from build123d import *

# Parameters (mm, degrees)
PAD_DEPTH          = 56
SKETCH005_R        = 1.25
POCKET_DEPTH       = 236.830052
POCKET_DEPTH_BACK  = 294.830052
POCKET001_DEPTH    = 237.830052
POLARPATTERN_COUNT = 6


with BuildPart() as part:
    # Sketch → Revolution002 (revolve)
    with BuildSketch(Plane.XZ):
        with BuildLine():
            Line((12, 0), (12, 58))
            Line((12, 58), (36.5, 58))
            Line((36.5, 55), (36.5, 58))
            Line((31, 55), (36.5, 55))
            Line((31, 4.25), (31, 55))
            Line((36.5, 4.25), (31, 4.25))
            Line((36.5, 1.25), (36.5, 4.25))
            Line((36.5, 1.25), (17, 1.25))
            Line((17, 1.25), (17, 0.5))
            ThreePointArc((16.5, 0), (16.853553, 0.146447), (17, 0.5))
            Line((16.5, 0), (12, 0))
        make_face()
    revolve(axis=Axis((0, 0, 0), (0, 0, 1)))

    # Sketch004 → Pad (new body)
    with BuildSketch(Plane.XY.offset(58)):
        with BuildLine():
            ThreePointArc((30.765894, -3.802601), (31, 0), (30.765894, 3.802601))
            ThreePointArc((30.765894, 3.802601), (30.872245, 3.491837), (31.094507, 3.25))
            Line((31.907923, 2.668318), (31.094507, 3.25))
            ThreePointArc((32.765894, 1), (32.538832, 1.938003), (31.907923, 2.668318))
            Line((32.765894, 1), (32.765894, -1))
            ThreePointArc((31.907923, -2.668318), (32.538832, -1.938003), (32.765894, -1))
            Line((31.907923, -2.668318), (31.094507, -3.25))
            ThreePointArc((31.094507, -3.25), (30.872245, -3.491837), (30.765894, -3.802601))
        make_face()
    pad = extrude(amount=-PAD_DEPTH)

    # Sketch005 → Pocket (cut, two sides)
    with BuildSketch(Plane.XY) as pocket_sk:
        with Locations((31.25, 0)):
            Circle(SKETCH005_R)
    pocket = extrude(amount=-POCKET_DEPTH, mode=Mode.SUBTRACT) + extrude(pocket_sk.sketch, amount=POCKET_DEPTH_BACK, mode=Mode.SUBTRACT)

    # Sketch006 → Pocket001 (cut, through all)
    with BuildSketch(Plane.XY.offset(57)):
        with BuildLine():
            ThreePointArc((15.210029, 5.719923), (14.056331, 8.153652), (12.516493, 10.363393))
            ThreePointArc((12.41083, 12.132293), (12.17453, 11.230572), (12.516493, 10.363393))
            Line((20.118158, 24.097608), (12.41083, 12.132293))
            ThreePointArc((23.174899, 24.466591), (21.559851, 25.000154), (20.118158, 24.097608))
            ThreePointArc((32.743937, 7.970232), (29.150669, 16.90942), (23.174899, 24.466591))
            ThreePointArc((30.906067, 5.5), (32.405281, 6.303385), (32.743937, 7.970232))
            Line((16.693075, 4.75), (30.906067, 5.5))
            ThreePointArc((15.210029, 5.719923), (15.793016, 4.992554), (16.693075, 4.75))
        make_face()
    pocket001 = extrude(amount=POCKET001_DEPTH, mode=Mode.SUBTRACT)

    # PolarPattern: Pad, Pocket, Pocket001 ×6 about axis
    polarpattern_axis = Axis((0, 0, 58), (0, 0, 1))
    for i in range(1, POLARPATTERN_COUNT):
        add(pad.rotate(polarpattern_axis, i * 360 / POLARPATTERN_COUNT))
        add(pocket.rotate(polarpattern_axis, i * 360 / POLARPATTERN_COUNT), mode=Mode.SUBTRACT)
        add(pocket001.rotate(polarpattern_axis, i * 360 / POLARPATTERN_COUNT), mode=Mode.SUBTRACT)


solid = part.part
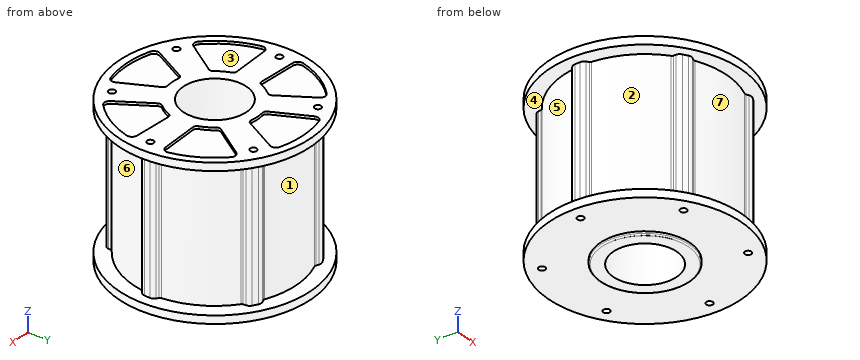
Read the model definition and answer for the solid it produces. Units are mm, in the model's axes. Face numbers are marked on the shaded views. A direction names the side the tool comes from. Coordinates: 2 decimals unless noted, no trailing zeros. Loops run counter-clockwise (first coordinate to the right, second up) from the corner with the lowest first, then second, coordinate; pieces in that order, holes last. Notation, with made-up numbers: (14.5, 14) - (58.5, 14) arc R7 ccw to (58.5, 18) - close; hole circle Ø6 at (45.25, -1). An arc over 180 degrees is marked (long way). Answer in a Markdown table with one row per item.
Q1. Straight lines are drawn through the part: line 1 along X through (y, z) = (-27, 39); line 2 along Z through (x, y) = (-21, -3); line 3 along Z through (x, y) = (18, 12). For each, find the intervals that lie inside material, in ascending order. Write a range as [from, to].
Here are the results:
| item | result |
|---|---|
| line 1 | x = [-18.07, -16.87], [-14.38, 14.38], [16.87, 18.07] |
| line 2 | z = [1.25, 58] |
| line 3 | z = [1.25, 57] |
Q2. The mould has two halves that part along X. Classify the marked faces 5, 6 and 7: pulls with the +X half, pulls with the -X half, needs draft (parallel to the pull), parting line crosses it, or undercut.
Here are the results:
| item | result |
|---|---|
| face 5 | pulls with the -X half |
| face 6 | pulls with the +X half |
| face 7 | undercut |
Q3. Given P1, Ø10, axis at y = 17.5, z = 37, coming from the +X side; P2, Ø1.5, axis at x = 31.25, y = 0, coming from the +Z side; P3, Ø2, axis at y = 0, z = 36, coming from the +X side; P4, Ø1, axis at x = 17, z = 18, coming from the +Y side, each flat-ended and moving along its own axis, determine where each tip first touches the part or whether it passes through.
Here are the results:
| item | result |
|---|---|
| P1 | stops at x = 28.37 |
| P2 | passes through |
| P3 | stops at x = 32.77 |
| P4 | stops at y = 28.31 |
Q4. Find section B-B on y = 0. Count the separate pieces of the cut face and the enclosed holes in it, plus the area to 3 significant figures.
Here are the results:
| item | result |
|---|---|
| separate pieces | 4 |
| enclosed holes | 0 |
| area | 2,130 mm^2 |
Q5. For the marked faces 1, 2, 3 and 4, determine the directions among +Z, -Z, +X, -X, +Y, -Y from which every point of the face is accessible in a straight line to the end or side of a thin tool.
Here are the results:
| item | result |
|---|---|
| face 1 | +Y |
| face 2 | -X, -Y |
| face 3 | +Z |
| face 4 | none |
Q6. Find section C-C on x = 25. Write down the section's boundary in (y, z).
Here are the results:
| item | result |
|---|---|
| outline | (-26.59, 1.25) - (26.59, 1.25) - (26.59, 4.25) - (18.33, 4.25) - (18.33, 55) - (26.59, 55) - (26.59, 58) - (22.6, 58) - (22.6, 57) - (5.19, 57) - (5.19, 58) - (-5.09, 58) - (-5.09, 57) - (-22.6, 57) - (-22.6, 58) - (-26.59, 58) - (-26.59, 55) - (-18.33, 55) - (-18.33, 4.25) - (-26.59, 4.25) - close |
Q7. Find section D-D on y = 20.5. Write down the section's boundary in (x, z).
Here are the results:
| item | result |
|---|---|
| outline | (-30.2, 1.25) - (30.2, 1.25) - (30.2, 4.25) - (23.25, 4.25) - (23.25, 55) - (30.2, 55) - (30.2, 58) - (26.75, 58) - (26.75, 57) - (17.8, 57) - (17.8, 58) - (6.1, 58) - (6.1, 57) - (-6.2, 57) - (-6.2, 58) - (-17.93, 58) - (-17.93, 57) - (-26.75, 57) - (-26.75, 58) - (-30.2, 58) - (-30.2, 55) - (-23.25, 55) - (-23.25, 4.25) - (-30.2, 4.25) - close |
